Check sheet for the drawn part. Datum: minimum x, y, z corner. Units: mm. A direction names the side the tool comes from. Give positions to 0.01 mm unless a question says otherwise; leave off trailing zeros. Write each loop counter-clockwise with the first axis right and the second up, starting at its lowest first coordinate (ties: lowest second). Pieces come first, ordered by that corner, then holes. Notation, with made-up numbers: (25, 1) -> (69, 1) arc R23 ccw to (69, 26) -> close; hole circle Ø9 at (59, 19). An arc over 180 degrees is marked (long way). Answer as CSV lines item,"result". Start each with the question number.
1) Mould release check, pull along Y, two halves, no side actions. Record for the marked faces 3, 4, 5 and 6: released by +Y, released by -Y, zero draft, split by the parting line, or undercut.
2) Material ranges on L1, parallel to X at y = 5.5, z = 9.75; L2, parallel to Y at x = 27.5, z = 4.5, recorded low to high.
3) Sectioned sample at C-C on z = 2. Record the cut outline in (x, y), and give its area (3 significant figures).
4) Tool access check on the marked faces 1 and 2. Record the directions out of +Z, -Z, +X, -X, +Y, -Y that give a thin tool (end or side, any length) a straight path to the whole face; none if there is none.
5) Sectioned sample at B-B on x = 17. Record the cut outline in (y, z).
6) Sectioned sample at A-A on y = 12.25. Record the cut outline in (x, z).
7) Gauge pin test, flat ends, axial feed: pin 1 Ø2.5 at (x, z) = (8, 4) entering from -Y; pin 2 Ø2 at (x, y) = (7, 8) entering from +Z. Record the tip position at first contact, or that the pin passes through.
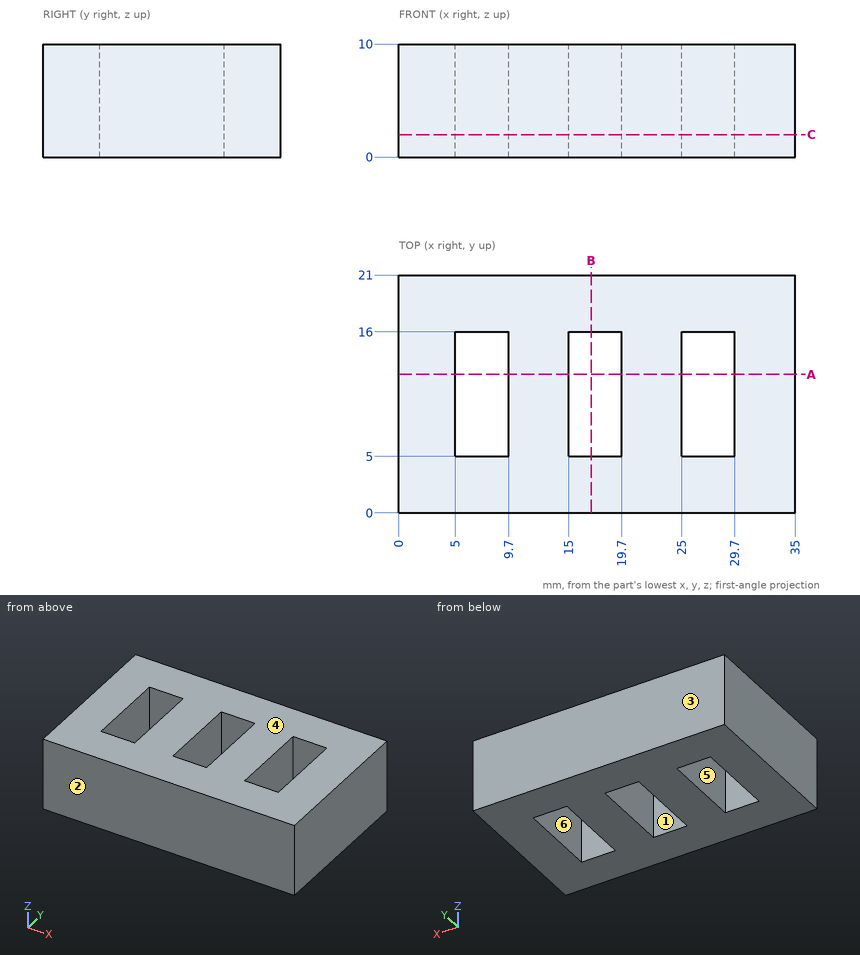
Ans:
1,face 3,"released by +Y"
1,face 4,"zero draft"
1,face 5,"undercut"
1,face 6,"undercut"
2,L1,"x = 0 to 5, 9.7 to 15, 19.7 to 25, 29.7 to 35"
2,L2,"y = 0 to 5, 16 to 21"
3,outline,"(0, 0) -> (35, 0) -> (35, 21) -> (0, 21) -> close; hole (5, 5) -> (9.7, 5) -> (9.7, 16) -> (5, 16) -> close; hole (15, 5) -> (19.7, 5) -> (19.7, 16) -> (15, 16) -> close; hole (25, 5) -> (29.7, 5) -> (29.7, 16) -> (25, 16) -> close"
3,area,"580 mm²"
4,face 1,"+Z, -Z"
4,face 2,"+Z, -Z, +X, -X, -Y"
5,outline,"(0, 0) -> (5, 0) -> (5, 10) -> (0, 10) -> close; (16, 0) -> (21, 0) -> (21, 10) -> (16, 10) -> close"
6,outline,"(0, 0) -> (5, 0) -> (5, 10) -> (0, 10) -> close; (9.7, 0) -> (15, 0) -> (15, 10) -> (9.7, 10) -> close; (19.7, 0) -> (25, 0) -> (25, 10) -> (19.7, 10) -> close; (29.7, 0) -> (35, 0) -> (35, 10) -> (29.7, 10) -> close"
7,pin 1,"stops at y = 0"
7,pin 2,"passes through"
